Geometry check sheet. Reference: drawing and pictorial views, mm from the part's lowest x, y, z. Round coordinates to 2 decimals unless told otherwise and drop trailing zeros. Order: outer loops, then holes, each group sorted by start corner. A loop starts at its lowest first (then second) coordinate and runs counter-clockwise, first axis right, second up.
(1) Thickness scan on probe 1 along X at (y, z) = (9, 14.5) (1 decimal); probe 2 along X at (y, z) = (6.25, 12.75) (1 decimal). Record the ranges inside material, lowest first.
(2) Mould release check, pull along Z, two halves, no side actions. Record for the marked faces 1, 2, 3 and 4: released by +Z, released by -Z, zero draft, split by the parting line, or undercut.
(3) Sectioned sample at A-A, the plane x = 17.5. Enter the section's corners in (y, z).
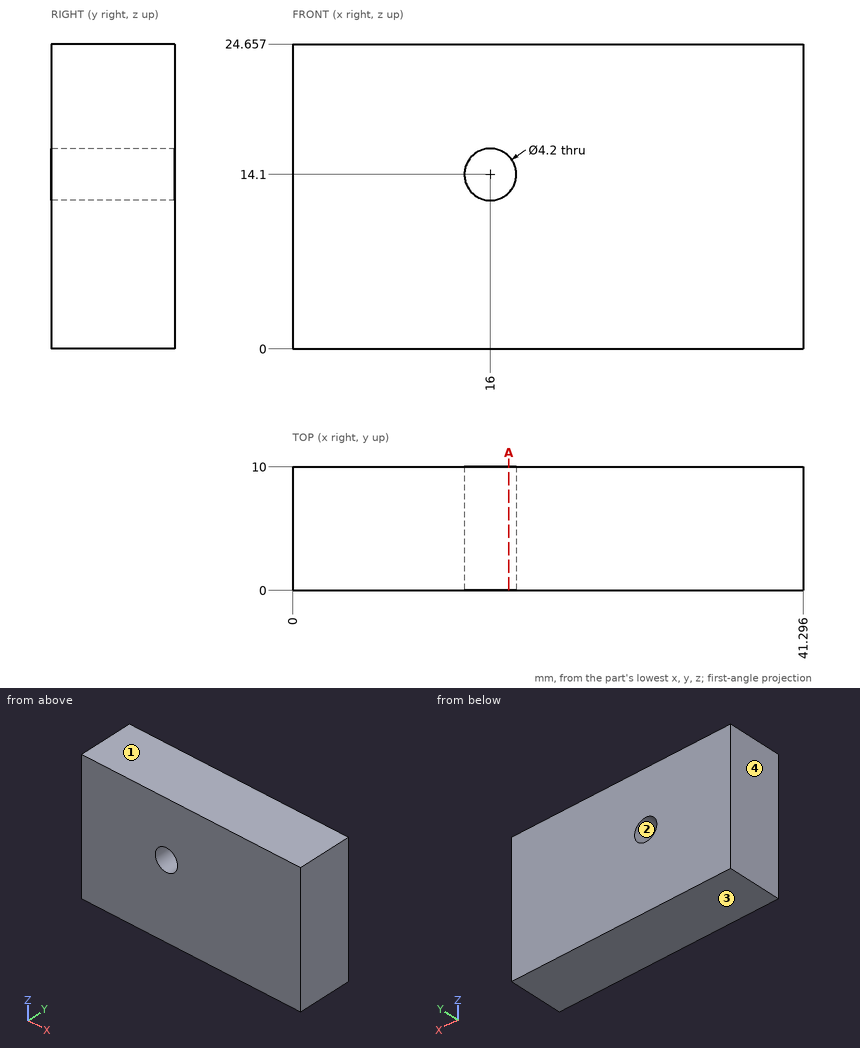
Derived:
1. probe 1: x = 0 to 13.9, 18.1 to 41.3
1. probe 2: x = 0 to 14.4, 17.6 to 41.3
2. face 1: released by +Z
2. face 2: undercut
2. face 3: released by -Z
2. face 4: zero draft
3. outline: (0, 0) - (10, 0) - (10, 12.63) - (0, 12.63) - close; (0, 15.57) - (10, 15.57) - (10, 24.66) - (0, 24.66) - close
